from build123d import *

# Parameters (mm, degrees)
SKETCH_4_W          = 36.75
SKETCH_4_H          = 10
SKETCH_4_R          = 1.5
EXTRUDE_1_DEPTH     = 5
SKETCH_5_W          = 36.75
SKETCH_5_H          = 5
EXTRUDE_2_DEPTH     = 20
EXTRUDE_START       = -10
SKETCH_5_2_W        = 36.75
SKETCH_5_2_H        = 5
EXTRUDE_3_DEPTH     = 20
SKETCH_6_R          = 1
CUT_EXTRUDE_1_DEPTH = 4
SKETCH_4_5_R        = 2.25
CUT_EXTRUDE_2_DEPTH = 2


with BuildPart() as part:
    # 草图4 → 凸台-拉伸1 (new body)
    with BuildSketch(Plane(origin=(0, 0, 0), x_dir=(1, 0, 0), z_dir=(0, 1, 0))):
        with Locations((-18.375, -5)):
            Rectangle(SKETCH_4_W, SKETCH_4_H)
        with Locations(Location((-31.75, -5, 0), (0, 0, 270))):
            Circle(SKETCH_4_R, mode=Mode.SUBTRACT)
        with Locations(Location((-10, -5, 0), (0, 0, 270))):
            Circle(SKETCH_4_R, mode=Mode.SUBTRACT)
    extrude(amount=EXTRUDE_1_DEPTH)

    # 草图5 → 凸台-拉伸2 (add)
    with BuildSketch(Plane.XY.offset(10)):
        with Locations((-18.375, 2.5)):
            Rectangle(SKETCH_5_W, SKETCH_5_H)
    extrude(amount=EXTRUDE_2_DEPTH)

    # 草图5<2> → 凸台-拉伸3 (add)
    with BuildSketch(Plane.XY.offset(10).offset(EXTRUDE_START)):
        with Locations((-18.375, 2.5)):
            Rectangle(SKETCH_5_2_W, SKETCH_5_2_H)
    extrude(amount=-EXTRUDE_3_DEPTH)

    # 草图6 → 切除-拉伸1 (cut)
    with BuildSketch(Plane.ZY.offset(36.75)):
        with Locations((-10, 2.5)):
            Circle(SKETCH_6_R)
        with Locations((20, 2.5)):
            Circle(SKETCH_6_R)
    extrude(amount=-CUT_EXTRUDE_1_DEPTH, mode=Mode.SUBTRACT)

    # 草图4<5> → 切除-拉伸2 (cut)
    with BuildSketch(Plane(origin=(0, 0, 0), x_dir=(1, 0, 0), z_dir=(0, 1, 0))):
        with Locations(Location((-31.75, -5, 0), (0, 0, 270))):
            Circle(SKETCH_4_5_R)
        with Locations(Location((-10, -5, 0), (0, 0, 270))):
            Circle(SKETCH_4_5_R)
    extrude(amount=CUT_EXTRUDE_2_DEPTH, mode=Mode.SUBTRACT)


solid = part.part
Check sheet for the modelled part. Datum: model origin and axes. Units: mm. A direction names the side the tool comes from. Round coordinates to 2 decimals unless told otherwise and drop trailing zeros. Order: outer loops, then holes, each group sorted by start corner. A loop starts at its lowest first (then second) coordinate and runs counter-clockwise, first axis right, second up.
(1) Cross-section at D-D, the plane z = -10. Enter the section's corners in (x, y), and give its area (3 significant figures).
(2) Scan lines: probe 1 along X at (y, z) = (2.9, 5); probe 2 along X at (y, z) = (1.45, 5); probe 3 along Y at (x, z) = (-33.7, -10). Record each from-to range of solid material in increasing order.
(3) Cross-section at A-A, the plane x = -10. Enter the section's corners in (y, z).
(4) Access from +Z, -Z, +X, -X, +Y, -Y to the whole of each face (thin tool, end or side, straight path). Record for faces 4 (the flat face through (-19, 0, 5)), 5 (the flat face through (-32.75, 3, -10)), 6 (the flat face through (-30, 2, 5)).
(5) Draft check along X on faces 1 (the flat face through (0, 2, 5)), 2 (the flat face through (-19, 5, 5)), 3 (the cylindrical face through (-8.103, 0.986, 6.21)). Enter one of: pulls with the +X half, pulls with the -X half, needs draft (parallel to the pull), parting line crosses it, or undercut.
(6) Go/stop test with flat-tipped pins: P1, Ø2, axis at x = -20, z = -3, coming from the -Y side; P2, Ø1.2, axis at y = 2.5, z = -10, coming from the -X side; P3, Ø3.5, axis at x = -32, z = 5, coming from the -Y side. Record where each tip stops, or that it passes through.
(7) Cross-section at C-C, the plane y = 2.5. Enter the section's corners in (x, z), and give its area (3 significant figures).
(8) Cross-section at B-B, the plane z = 5. Enter the section's corners in (x, y).
Check sheet entries:
1. outline: (-36.75, 0) - (0, 0) - (0, 5) - (-36.75, 5) - (-36.75, 3.5) - (-32.75, 3.5) - (-32.75, 1.5) - (-36.75, 1.5) - close
1. area: 176 mm2
2. probe 1: x = -36.75 to -33.25, -30.25 to -11.5, -8.5 to 0
2. probe 2: x = -36.75 to -34, -29.5 to -12.25, -7.75 to 0
2. probe 3: y = 0 to 1.5, 3.5 to 5
3. outline: (0, -20) - (5, -20) - (5, 3.5) - (2, 3.5) - (2, 2.75) - (0, 2.75) - close; (0, 7.25) - (2, 7.25) - (2, 6.5) - (5, 6.5) - (5, 30) - (0, 30) - close
4. face 4: +Z, -Z, +X, -X, -Y
4. face 5: -X
4. face 6: -Y
5. face 1: pulls with the +X half
5. face 2: needs draft
5. face 3: undercut
6. P1: stops at y = 0
6. P2: stops at x = -32.75
6. P3: stops at y = 2
7. outline: (-36.75, -20) - (0, -20) - (0, 30) - (-36.75, 30) - (-36.75, 21) - (-32.75, 21) - (-32.75, 19) - (-36.75, 19) - (-36.75, -9) - (-32.75, -9) - (-32.75, -11) - (-36.75, -11) - close; hole circle Ø3 at (-31.75, 5); hole circle Ø3 at (-10, 5)
7. area: 1,810 mm2
8. outline: (-36.75, 0) - (-34, 0) - (-34, 2) - (-33.25, 2) - (-33.25, 5) - (-36.75, 5) - close; (-30.25, 2) - (-29.5, 2) - (-29.5, 0) - (-12.25, 0) - (-12.25, 2) - (-11.5, 2) - (-11.5, 5) - (-30.25, 5) - close; (-8.5, 2) - (-7.75, 2) - (-7.75, 0) - (0, 0) - (0, 5) - (-8.5, 5) - close
